Autodesk Inventor part; units mm, degrees
ref_plane "IDS_WORKPLANE{1}" through (-3.8354, 0, 0) normal (-1, 0, 0) x (0, 0, -1)
ref_plane "Work Plane3" through (7, 0, 0) normal (0, 0, -1) x (1, 0, 0)
ref_plane "YZ Plane" through (0, 0, 0) normal (1, 0, 0) x (0, 1, 0)
sketch "Sketch1" plane through (0, 0, 0) normal (0, 0, 1) x (1, 0, 0)
  line L0 (-0.7874, 5.2578) -> (-0.7874, 0)
  line L1 (-0.7874, 0) -> (31.75, 0)
  line L2 (31.75, 0) -> (31.75, 2.413)
  line L3 (31.75, 2.413) -> (0, 2.413)
  line L4 (0, 2.413) -> (0, 5.2578)
  line L5 (-7.2949, 0) -> (38.2575, 0)
  line L6 (0, -1.0516) -> (0, 6.3094)
  line L7 (0, 5.2578) -> (-0.7874, 5.2578)
  dimension "d1" = 0.7874
  dimension "d2" = 4.826
  dimension "d3" = 31.75
  dimension "d22" = 10.5156
revolve "Body" add sketch "Sketch1" angle 360 about axis through (-0.7874, 0, 0) along (1, 0, 0)
sketch "Sketch2" plane through (-0.7874, 0, 0) normal (-1, 0, 0) x (0, 0, 1)
  line L0 (0, 4.5754) -> (3.9624, 2.2877)
  line L1 (3.9624, 2.2877) -> (3.9624, -2.2877)
  line L2 (3.9624, -2.2877) -> (0, -4.5754)
  line L3 (0, -4.5754) -> (-3.9624, -2.2877)
  line L4 (-3.9624, -2.2877) -> (-3.9624, 2.2877)
  line L5 (-3.9624, 2.2877) -> (0, 4.5754)
  circle A0 centre (0, 0) radius 5.2578
  dimension "d11" = 7.9248
extrude "Head" add sketch "Sketch2" along normal blind 3.048 contours L0 L1 L2 L3 L4 L5
ref_plane "IDS_WORKPLANE{1}" through (-3.8354, 0, 0) normal (-1, 0, 0) x (0, 0, -1)
sketch "Sketch3" plane through (-3.8354, 0, 0) normal (-1, 0, 0) x (0, 0, -1)
  circle A0 centre (0, 0) radius 3.1699
  point P0 (0, 0)
  dimension "d15" = 6.3398
extrude "Indent" cut sketch "Sketch3" against normal blind 0.3048
thread "Thread"
sketch "Sketch4" plane through (0, 0, 0) normal (0, 0, 1) x (1, 0, 0)
  line L0 (-3.8354, 3.9624) -> (-3.8354, 4.5754)
  line L1 (-3.8354, 4.5754) -> (-3.3472, 4.5754)
  line L2 (-3.8354, 4.5754) -> (-3.8354, 2.2877)
  line L3 (-4.9666, 0) -> (2.8908, 0)
  line L4 (-0.7874, 4.5754) -> (-3.8354, 4.5754)
  arc A0 (-3.3472, 4.5754) -> (-3.8354, 3.9624) centre (1.7683, 0) ccw
  dimension "d21" = 7.9248
  dimension "d23" = 6.8631
revolve "Chamfer1" cut sketch "Sketch4" angle 360 about axis through (-10, 0, 0) along (1, 0, 0)
chamfer "Chamfer2" distance 0.5334 distance2 3.7084 1 edges at (31.75, -2.413, 0) measured on face at (31.75, 0.5787, 0.3409)
ref_plane "Work Plane3" through (7, 0, 0) normal (0, 0, -1) x (1, 0, 0)
equation "\"d1\" = SD"
equation "\"d2\" = NND"
equation "\"d3\" = NLG"
equation "\"d22\" = SD2"
equation "\"d11\" = SW"
equation "\"d12\" = KOH"
equation "\"d15\" = SD3"
equation "\"d16\" = SB"
equation "\"d21\" = SW"
equation "\"d23\" = 0.866025 * SW"
equation "\"d6\" = GEL"
equation "\"d19\" = -0.5 * GD2 + 0.5 * NND"
equation "\"d20\" = SPTZ"
equation "\"NLG\" = 31.75"
equation "\"NND\" = 4.826"
equation "\"KOH\" = 3.048"
equation "\"GEL\" = 31.75"
equation "\"SW\" = 7.9248"
equation "\"GD2\" = 3.7592"
equation "\"SPTZ\" = 3.7084"
equation "\"SD3\" = 0.8 * SW"
equation "\"SB\" = 0.1 * KOH"
equation "\"SD2\" = 10.5156"
equation "\"SD\" = 0.7874"
equation "\"GD1\" = 3.7592"
equation "\"THREADDIA\" = 4.826"
equation "\"TOA\" = 30deg"
equation "\"E0\" = 9.15077"
properties part number "am-1266" material "Steel, Mild"
Read the model definition and answer for the solid it produces. Units are mm, in the model's axes. A direction names the side the tool comes from. Round coordinates to 2 decimals unless told otherwise and drop trailing zeros. Order: outer loops, then holes, each group sorted by start corner. A loop starts at its lowest first (then second) coordinate and runs counter-clockwise, first axis right, second up. Notation, with made-up numbers: (68.25, 63) - (115.25, 63) arc R13 ccw to (115.25, 80) - close; hole circle Ø10 at (12.5, -14). An arc over 180 degrees is marked (long way). Use one line per item in the form item = value. Start each with the question number.
(1) The part is cut by section A-A (x = 16). Give the vertices of the cut face in (y, z), then the cut area to 3 significant figures.
(2) For faces 1 (the face through (-2.29, -3.45, -1.95)), 2 (the face through (-2, 0, -3.962)), 3 (the face through (-2, 0, 3.962)), determine the directions among +Z, -Z, +X, -X, +Y, -Y from which every point of the face is accessible in a straight line to the end or side of a thin tool.
(3) Flat-ended cylindrical pins translate along their axes: pin 1 Ø1.9 at (y, z) = (-1, 0) entering from -X; pin 2 Ø0.9 at (x, y) = (-2.5, 0) entering from +Z; pin 3 Ø6 at (x, y) = (11, 0) entering from -Z; pin 4 Ø1.5 at (x, z) = (25.5, -3.5) entering from +Y (3 decimals). Find the tip coordinate at first contact, or state that the pin passes through.
(4) Find the intervals of material crossed by line 1 along Z through (x, y) = (-3.65, 0); line 2 along X through (y, z) = (4.75, 0); line 3 along X through (y, z) = (0, 0), in increasing order. Write a range as from..to.
(5) The part is cut by section B-B (z = 4.75). Give the vertices of the cut face in (x, y), then the cut area to 3 significant figures.
(6) Determine the mould class of faces 4 (the face through (-3.531, 0, 0)), 5 (the face through (31.75, 0, 0)), 6 (the face through (-2.29, 3.416, -2.009)) for opening direction Z: +Z half, -Z half, draft (parallel to the pull), parting line (faces both ways), or undercut.
Checked values:
q1.outline = circle Ø4.83 at (0, 0)
q1.area = 18.3 mm^2
q2.face_1 = -Z, -X, -Y
q2.face_2 = -Z, -X, +Y, -Y
q2.face_3 = +Z, -X, +Y, -Y
q3.pin_1 = -3.53
q3.pin_2 = 3.96
q3.pin_3 = -2.41
q3.pin_4 = through
q4.line_1 = -3.96..-3.17, 3.17..3.96
q4.line_2 = -0.79..0
q4.line_3 = -3.53..31.75
q5.outline = (-0.79, -2.25) - (0, -2.25) - (0, 2.25) - (-0.79, 2.25) - close
q5.area = 3.55 mm^2
q6.face_4 = undercut
q6.face_5 = draft
q6.face_6 = -Z half
